```python
from build123d import *

# Parameters (mm, degrees)
F1_DEPTH = 110
F2_W     = 15
F2_H     = 40
F3_DEPTH = 3


# Not quite as in the source:
# - a feature names something its author has since deleted; it is built from what else it names


with BuildPart() as f1:
    # F0 (on Front) → F1 (new body)
    with BuildSketch(Plane.XZ):
        Polygon((0, 5), (0, 0), (75, 0), (75, 52), (73, 52), (73, 50), (71, 50), (71, 15.0446529165), (67, 15.0446529165), (60.9553470835, 9), (60.9553470835, 5), align=None)
    extrude(amount=F1_DEPTH)

    # F2 (on face) → F3 (cut)
    with BuildSketch(Plane.XY.offset(5)):
        with Locations((42.5, -45)):
            Rectangle(F2_W, F2_H)
    extrude(amount=-F3_DEPTH, mode=Mode.SUBTRACT)

    # F4: F1 across plane


with BuildPart() as f1_1:
    add(f1.part)
    add(f1.part.mirror(Plane.YZ))


solid = f1_1.part
```
Read the model definition and answer for the solid it produces. Units are mm, in the model's axes. A direction names the side the tool comes from. Round coordinates to 2 decimals unless told otherwise and drop trailing zeros. Write each loop counter-clockwise with the first axis right and the second up, starting at its lowest first coordinate (ties: lowest second). Pieces come first, ordered by that corner, then holes. Notation, with made-up numbers: (62.25, 44.25) -> (95.25, 44.25) arc R35 cw to (95.25, 79.25) -> close; hole circle Ø11 at (29.5, 14). An arc over 180 degrees is marked (long way). Answer in a Markdown table with one row per item. Add a question column.
1) Given P1, Ø16.5, axis at x = 45.5, y = -40.5, coming from the +Z side; P2, Ø1.6, axis at x = -71.5, y = -33.5, coming from the +Z side; P3, Ø1.2, axis at x = 69.5, y = -51, coming from the +Z side, each flat-ended and moving along its own axis, determine where each tip first touches the part or whether it passes through.
2) Find section C-C, the plane x = 25. Determine the outline of the cut face in (y, z), and give its area (3 significant figures).
3) Find section B-B, the plane y = -14.5. Determine the outline of the cut face in (x, z).
4) Find section D-D, the plane y = -40. Determine the outline of the cut face in (x, z), and give its area (3 significant figures).
5) Find section A-A, the plane z = 43. Determine the outline of the cut face in (x, y), and give its area (3 significant figures).
6) Determine the mould class of faces 4 (the face through (69, -54, 15.045)), 5 (the face through (-75, -54, 26)), 6 (the face through (42, -65, 4)), 7 (the face through (1, -54, 0)) for opening direction X: pulls with the +X half, pulls with the -X half, needs draft (parallel to the pull), parting line crosses it, or undercut.
7) Consider line 1 (X direction, y = -97, z = 41.5); line 2 (Z direction, x = -55, y = -86); line 3 (X direction, y = -101.5, z = 12). Determine where each line is inside the solid, lowest interval first.
8) Which of the six approach directions +Z, -Z, +X, -X, +Y, -Y give full straight-line access (tool end or side, diameter ignored) to faces 1 (the face through (-69, -54, 15.045)), 2 (the face through (0, 0, 3)), 3 (the face through (-42, -25, 4))?
Findings below:
| question | item | result |
|---|---|---|
| 1 | P1 | z = 5 |
| 1 | P2 | z = 50 |
| 1 | P3 | z = 15.04 |
| 2 | outline | (-110, 0) -> (0, 0) -> (0, 5) -> (-110, 5) -> close |
| 2 | area | 550 mm² |
| 3 | outline | (-75, 0) -> (75, 0) -> (75, 52) -> (73, 52) -> (73, 50) -> (71, 50) -> (71, 15.04) -> (67, 15.04) -> (60.96, 9) -> (60.96, 5) -> (-60.96, 5) -> (-60.96, 9) -> (-67, 15.04) -> (-71, 15.04) -> (-71, 50) -> (-73, 50) -> (-73, 52) -> (-75, 52) -> close |
| 4 | outline | (-75, 0) -> (75, 0) -> (75, 52) -> (73, 52) -> (73, 50) -> (71, 50) -> (71, 15.04) -> (67, 15.04) -> (60.96, 9) -> (60.96, 5) -> (50, 5) -> (50, 2) -> (35, 2) -> (35, 5) -> (-35, 5) -> (-35, 2) -> (-50, 2) -> (-50, 5) -> (-60.96, 5) -> (-60.96, 9) -> (-67, 15.04) -> (-71, 15.04) -> (-71, 50) -> (-73, 50) -> (-73, 52) -> (-75, 52) -> close |
| 4 | area | 1,190 mm² |
| 5 | outline | (-75, -110) -> (-71, -110) -> (-71, 0) -> (-75, 0) -> close; (71, -110) -> (75, -110) -> (75, 0) -> (71, 0) -> close |
| 5 | area | 880 mm² |
| 6 | face 4 | undercut |
| 6 | face 5 | pulls with the -X half |
| 6 | face 6 | undercut |
| 6 | face 7 | needs draft |
| 7 | line 1 | -75 to -71, 71 to 75 |
| 7 | line 2 | 0 to 5 |
| 7 | line 3 | -75 to -63.96, 63.96 to 75 |
| 8 | face 1 | +Z, +Y, -Y |
| 8 | face 2 | +Z, -Z, +X, -X, +Y |
| 8 | face 3 | +Z |
